Read the model definition and answer for the solid it produces. Units are mm, in the model's axes. Face numbers are marked on the shaded views. Give positions to 0.01 mm unless a question says otherwise; leave off trailing zeros. Order: outer loops, then holes, each group sorted by start corner. A loop starts at its lowest first (then second) coordinate and runs counter-clockwise, first axis right, second up.
Item 1: A cutting plane is placed at A-A (z = 0). Write down the section's boundary in (x, y).
Item 2: Find the intervals of material crossed by line 1 along Y through (x, z) = (-10, -3.5); line 2 along Y through (x, z) = (-4, 10.5); line 3 along Z through (x, y) = (-6, 4.5), in increasing order.
Item 3: A cutting plane is placed at D-D (x = -10.5). Write down the section's boundary in (y, z), plus the area to 3 significant figures.
Item 4: The mould has two halves that part along Z. Classify the marked faces 1, 2 and 3: +Z half, -Z half, draft (parallel to the pull), parting line (faces both ways), or undercut.
Item 5: Given pin 1 Ø1 at (y, z) = (4, -11.5) entering from -X; pin 2 Ø1.5 at (x, z) = (2.5, 4) entering from -Y; pin 3 Ø4 at (x, y) = (11, 1.5) entering from -Z; pin 4 Ø4 at (x, y) = (-6.5, 5.5) entering from +Z, each flat-ended and moving along its own axis, determine where each tip first touches the part or whether it passes through.
Item 6: A cutting plane is placed at C-C (z = 6.5). Write down the section's boundary in (x, y), plus the area to 3 significant figures.
Item 7: A cutting plane is placed at B-B (x = 0). Write down the section's boundary in (y, z).
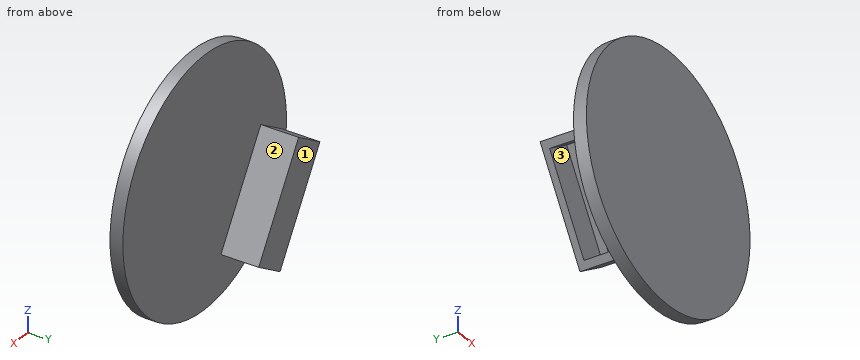
from build123d import *

# Parameters (mm, degrees)
SKETCH1_R           = 16.3
BOSS_EXTRUDE1_DEPTH = 1.7
BOSS_EXTRUDE2_DEPTH = 5
SKETCH3_W           = 12.912487974
SKETCH3_H           = 3.215299838
CUT_EXTRUDE1_DEPTH  = 4


with BuildPart() as part:
    # Sketch1 → Boss-Extrude1 (new body)
    with BuildSketch(Plane(origin=(0, 0, 0), x_dir=(1, 0, 0), z_dir=(0, 1, 0))):
        with Locations(Location((0, 0, 0), (0, 0, 270))):
            Circle(SKETCH1_R)
    extrude(amount=BOSS_EXTRUDE1_DEPTH)

    # Sketch2 → Boss-Extrude2 (add)
    with BuildSketch(Plane(origin=(0, 1.7, 0), x_dir=(1, 0, 0), z_dir=(0, 1, 0))):
        Polygon((-7.474254816, 13.514270788), (-15.42304378, 0.793549346), (-11.182803299, -1.856046975), (-3.234014336, 10.864674467), align=None)
    extrude(amount=BOSS_EXTRUDE2_DEPTH)

    # Sketch3 → Cut-Extrude1 (cut)
    with BuildSketch(Plane(origin=(-11.448649298, 0, -7.153910067), x_dir=(-0.5299192642332052, 0, 0.8480480961564258), z_dir=(-0.8480480961564258, 0, -0.5299192642332052))):
        with Locations((0, 4.2)):
            Rectangle(SKETCH3_W, SKETCH3_H)
    extrude(amount=-CUT_EXTRUDE1_DEPTH, mode=Mode.SUBTRACT)


solid = part.part
Response values:
1. outline: (-16.3, 0) - (16.3, 0) - (16.3, 1.7) - (-10.02, 1.7) - (-10.02, 6.7) - (-14.15, 6.7) - (-14.15, 1.7) - (-16.3, 1.7) - close; hole (-12.18, 2.59) - (-11.2, 2.59) - (-11.2, 5.81) - (-12.18, 5.81) - close
2. line 1: y = 0 to 2.59, 5.81 to 6.7
2. line 2: y = 0 to 1.7
2. line 3: z = -12.59 to -11.36, -8.33 to -6.44
3. outline: (0, -12.47) - (1.7, -12.47) - (1.7, -8.67) - (2.59, -8.67) - (2.59, -1.12) - (5.81, -1.12) - (5.81, -8.67) - (6.7, -8.67) - (6.7, 0.76) - (1.7, 0.76) - (1.7, 12.47) - (0, 12.47) - close
3. area: 65.3 mm2
4. face 1: draft
4. face 2: +Z half
4. face 3: undercut
5. pin 1: stops at x = -7.02
5. pin 2: stops at y = 0
5. pin 3: stops at z = -13.59
5. pin 4: stops at z = -2.44
6. outline: (-14.95, 0) - (14.95, 0) - (14.95, 1.7) - (-14.95, 1.7) - close
6. area: 50.8 mm2
7. outline: (0, -16.3) - (1.7, -16.3) - (1.7, 16.3) - (0, 16.3) - close
